Build history of the part. All positions in model axes, mm. Face numbers are marked on the shaded views. A direction names the side the tool comes from. Give positions to 0.01 mm unless a question says otherwise; leave off trailing zeros. Write each loop counter-clockwise with the first axis right and the second up, starting at its lowest first coordinate (ties: lowest second). Pieces come first, ordered by that corner, then holes. Notation, with made-up numbers: (17, 8) -> (50, 8) arc R28 cw to (50, 43) -> close; hole circle Ø4 at (-4, 50.5). An arc over 180 degrees is marked (long way). Put each result on its own line as item: value.
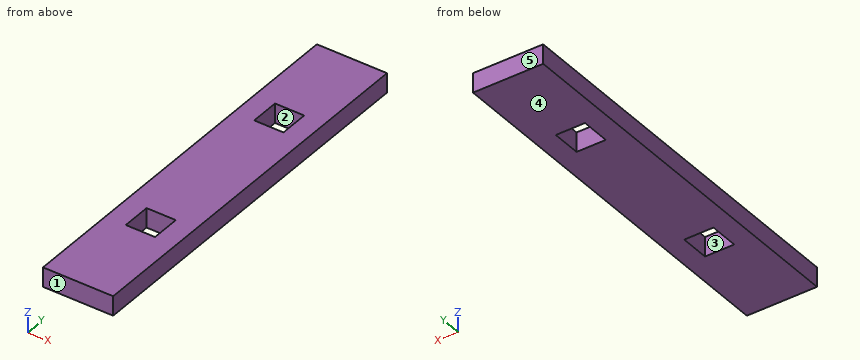
Autodesk Inventor part; units mm, degrees
ref_plane "YZ Plane" through (0, 0, 0) normal (1, 0, 0) x (0, 1, 0)
ref_plane "XZ Plane" through (0, 0, 0) normal (0, 1, 0) x (-1, 0, 0)
ref_plane "XY Plane" through (0, 0, 0) normal (0, 0, 1) x (1, 0, 0)
sketch "Sketch1" plane through (0, 0, 0) normal (0, 0, 1) x (1, 0, 0)
  line L0 (0, 0) -> (22.86, 0)
  line L1 (22.86, 0) -> (22.86, 125.5522)
  line L2 (22.86, 125.5522) -> (0, 125.5522)
  line L3 (0, 125.5522) -> (0, 0)
  line L4 (0, 62.7761) -> (22.86, 62.7761) construction
  line L5 (11.43, 96.9772) -> (16.1925, 96.9772)
  line L6 (16.1925, 96.9772) -> (16.1925, 87.4522)
  line L7 (16.1925, 87.4522) -> (6.6675, 87.4522)
  line L8 (6.6675, 87.4522) -> (6.6675, 96.9772)
  line L9 (6.6675, 96.9772) -> (11.43, 96.9772)
  line L10 (11.43, 28.575) -> (16.1925, 28.575)
  line L11 (16.1925, 28.575) -> (16.1925, 38.1)
  line L12 (16.1925, 38.1) -> (6.6675, 38.1)
  line L13 (6.6675, 38.1) -> (6.6675, 28.575)
  line L14 (6.6675, 28.575) -> (11.43, 28.575)
  dimension "d0" = 22.86
  dimension "d1" = 125.5522
  dimension "d13" = 4.7625
  dimension "d14" = 9.525
  dimension "d15" = 9.525
  dimension "d16" = 28.575
  dimension "d17" = 6.6675
extrude "Extrusion2" add sketch "Sketch1" along normal blind 6.35
properties part number "HopperSupportRod_v1"
1) Slice it at B-B (x = 12). Write the cut outline in (y, z) (3 decimals), plus the area to 3 significant figures.
Filled sheet:
outline: (0, 0) -> (28.575, 0) -> (28.575, 6.35) -> (0, 6.35) -> close; (38.1, 0) -> (87.452, 0) -> (87.452, 6.35) -> (38.1, 6.35) -> close; (96.977, 0) -> (125.552, 0) -> (125.552, 6.35) -> (96.977, 6.35) -> close
area: 676 mm2
2) Tool access for the marked faces 1 and 2: list every direction of +Z, -Z, +X, -X, +Y, -Y with a clear straight run to the whole face (end or side of a thin tool).
Filled sheet:
face 1: +Z, -Z, +X, -X, -Y
face 2: +Z, -Z
3) Pull direction Y, two halves, no side cores. Call the marked faces 3, 4 and 5: released by +Y, released by -Y, zero draft, split by the parting line, or undercut.
Filled sheet:
face 3: undercut
face 4: zero draft
face 5: released by +Y
4) Slice it at A-A (z = 1). Write the cut outline in (x, y) (1 decimal).
Filled sheet:
outline: (0, 0) -> (22.9, 0) -> (22.9, 125.6) -> (0, 125.6) -> close; hole (6.7, 28.6) -> (16.2, 28.6) -> (16.2, 38.1) -> (6.7, 38.1) -> close; hole (6.7, 87.5) -> (16.2, 87.5) -> (16.2, 97) -> (6.7, 97) -> close
5) Wall check: L1, parallel to Y at x = 10, z = 2.5 (3 decimals); L2, parallel to X at y = 94.5, z = 0.5. Give the ranges that are in metal, low to high.
Filled sheet:
L1: 0 to 28.575, 38.1 to 87.452, 96.977 to 125.552
L2: 0 to 6.67, 16.19 to 22.86
